```python
from build123d import *

# Parameters (mm, degrees)
SKETCH1_W           = 110
SKETCH1_H           = 70
BOSS_EXTRUDE1_DEPTH = 3
SKETCH2_R           = 2
SKETCH2_R_2         = 2.5
CUT_EXTRUDE1_DEPTH  = 5
SKETCH3_R           = 9.5
SKETCH3_R_2         = 2
CUT_EXTRUDE3_DEPTH  = 9


with BuildPart() as part:
    # Sketch1 → Boss-Extrude1 (new body)
    with BuildSketch(Plane.XY):
        with Locations((55, 35)):
            Rectangle(SKETCH1_W, SKETCH1_H)
    extrude(amount=BOSS_EXTRUDE1_DEPTH)

    # Sketch2 → Cut-Extrude1 (cut)
    with BuildSketch(Plane.XY.offset(3)):
        with Locations((5, 64)):
            Circle(SKETCH2_R)
        with Locations((5, 6)):
            Circle(SKETCH2_R)
        with Locations((105, 64)):
            Circle(SKETCH2_R_2)
        with Locations((105, 6)):
            Circle(SKETCH2_R_2)
        with Locations((5, 35)):
            Circle(SKETCH2_R)
    extrude(amount=-CUT_EXTRUDE1_DEPTH, mode=Mode.SUBTRACT)

    # Sketch3 → Cut-Extrude3 (cut)
    with BuildSketch(Plane.XY.offset(3)):
        with Locations((60, 35)):
            Circle(SKETCH3_R)
        with Locations((49, 49)):
            Circle(SKETCH3_R_2)
        with Locations((89, 49)):
            Circle(SKETCH3_R_2)
        with Locations(Location((89, 21, 0), (0, 0, 180))):
            Circle(SKETCH3_R_2)
        with Locations(Location((49, 21, 0), (0, 0, 180))):
            Circle(SKETCH3_R_2)
    extrude(amount=-CUT_EXTRUDE3_DEPTH, mode=Mode.SUBTRACT)


solid = part.part
```
Can you work these out from the model? Positions are in its coordinate system, mm. Give positions to 0.01 mm unless a question says otherwise; leave off trailing zeros. Write each loop counter-clockwise with the first axis right and the second up, starting at its lowest first coordinate (ties: lowest second). Pieces come first, ordered by that corner, then holes. Notation, with made-up numbers: (-24.5, 75.25) - (14.5, 75.25) arc R25 ccw to (14.5, 110.25) - close; hole circle Ø4 at (87.5, -33.5). An arc over 180 degrees is marked (long way). Write item = value, one per line. Start each with the question number.
1. Imagine slicing it at D-D (x = 60). Please give me the cut outline in (y, z).
2. Imagine slicing it at C-C (z = 1.25). Count the separate pieces of the cut face and the enclosed holes in it, and give its area (3 significant figures).
3. Thinking about a two-plate mould opening in X: for faces 1 (the face through (54, 0, 1)), 2 (the face through (49, 19, 2)), 3 (the face through (0, 35, 1)), 4 (the face through (107.385, 6.751, 1.521)), which applies, released by +X, released by -X, zero draft, split by the parting line, or undercut?
4. Imagine slicing it at A-A (y = 35). Please give me the cut outline in (x, z), and give its area (3 significant figures).
5. Please list where these lines run through material, in increasing order: line 1 (Y direction, x = 105, z = 1.1); line 2 (X direction, y = 21, z = 1.6); line 3 (Y direction, x = 60, z = 0.6).
6. Imagine slicing it at B-B (x = 49). Please give me the cut outline in (y, z).
Worked answers:
q1.outline = (0, 0) - (25.5, 0) - (25.5, 3) - (0, 3) - close; (44.5, 0) - (70, 0) - (70, 3) - (44.5, 3) - close
q2.separate_pieces = 1
q2.enclosed_holes = 10
q2.area = 7,290 mm2
q3.face_1 = zero draft
q3.face_2 = undercut
q3.face_3 = released by -X
q3.face_4 = undercut
q4.outline = (0, 0) - (3, 0) - (3, 3) - (0, 3) - close; (7, 0) - (50.5, 0) - (50.5, 3) - (7, 3) - close; (69.5, 0) - (110, 0) - (110, 3) - (69.5, 3) - close
q4.area = 261 mm2
q5.line_1 = 0 to 3.5, 8.5 to 61.5, 66.5 to 70
q5.line_2 = 0 to 47, 51 to 87, 91 to 110
q5.line_3 = 0 to 25.5, 44.5 to 70
q6.outline = (0, 0) - (19, 0) - (19, 3) - (0, 3) - close; (23, 0) - (47, 0) - (47, 3) - (23, 3) - close; (51, 0) - (70, 0) - (70, 3) - (51, 3) - close
